Study the drawing (mm; zero at the part's minimum x, y, z) and answer. A direction names the side the tool comes from. Give positions to 0.01 mm unless a question says otherwise; leave off trailing zeros. Order: outer loops, then holes, each group sorted by start corner. A loop starts at its lowest first (then second) coordinate and runs counter-clockwise, first axis right, second up. Notation, with made-up numbers: (84.25, 41.5) - (134.25, 41.5) arc R8 ccw to (134.25, 46.5) - close; hole circle Ø4 at (53.25, 5.25). An arc over 180 degrees is marked (long way). Return JSON: item names as keys, results as strings.
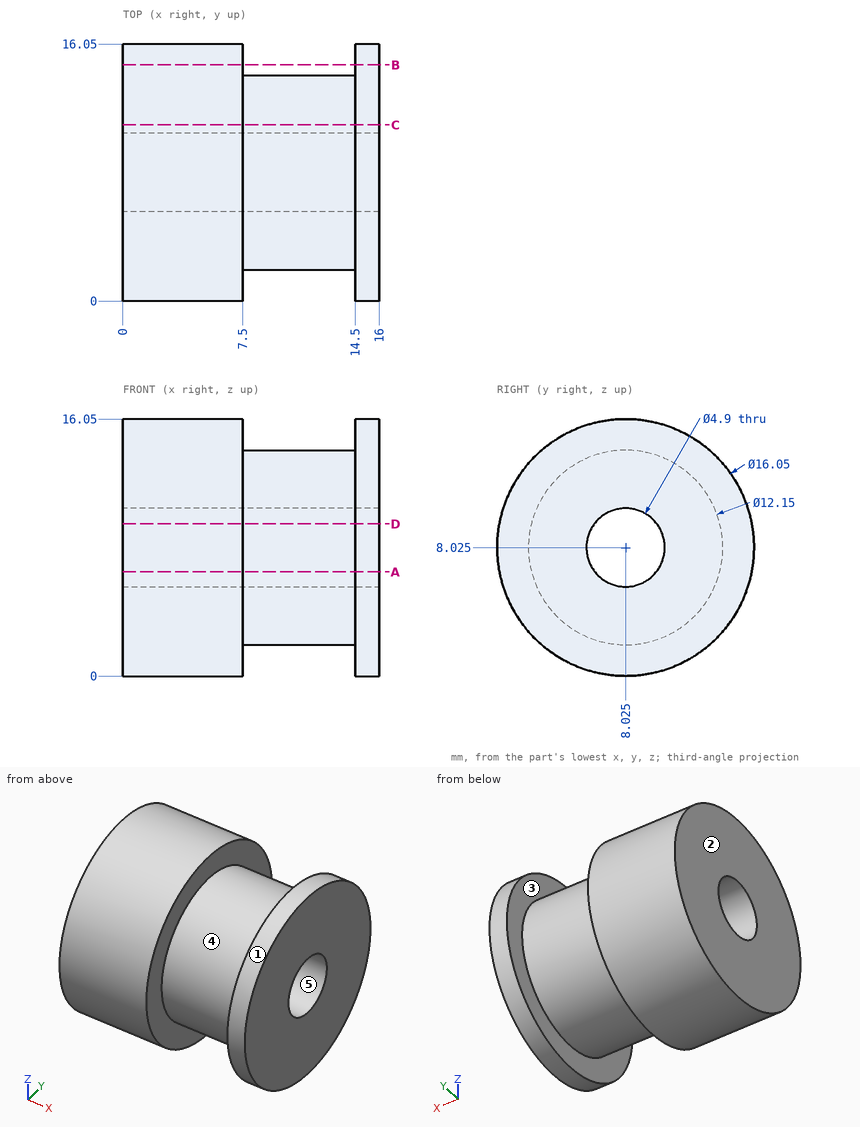
Q1. A cutting plane is placed at A-A (z = 6.5). Write down the section's boundary in (x, y).
Values:
{"outline": "(0, 0.15) - (7.5, 0.15) - (7.5, 2.14) - (14.5, 2.14) - (14.5, 0.15) - (16, 0.15) - (16, 6.11) - (0, 6.11) - close; (0, 9.94) - (16, 9.94) - (16, 15.9) - (14.5, 15.9) - (14.5, 13.91) - (7.5, 13.91) - (7.5, 15.9) - (0, 15.9) - close"}
Q2. A cutting plane is placed at C-C (y = 11). Write down the section's boundary in (x, z).
Values:
{"outline": "(0, 0.57) - (7.5, 0.57) - (7.5, 2.73) - (14.5, 2.73) - (14.5, 0.57) - (16, 0.57) - (16, 15.48) - (14.5, 15.48) - (14.5, 13.32) - (7.5, 13.32) - (7.5, 15.48) - (0, 15.48) - close"}
Q3. Determine the mould class of the marked faces 1, 2 and 3 for opening direction X: released by +X, released by -X, zero draft, split by the parting line, or undercut.
Values:
{"face 1": "zero draft", "face 2": "released by -X", "face 3": "undercut"}
Q4. A cutting plane is placed at B-B (y = 14.75). Write down the section's boundary in (x, z).
Values:
{"outline": "(0, 3.65) - (7.5, 3.65) - (7.5, 12.4) - (0, 12.4) - close; (14.5, 3.65) - (16, 3.65) - (16, 12.4) - (14.5, 12.4) - close"}
Q5. Given pin 1 (1 mm diameter, centred on x = 6.5, y = 2.5, fed in from -Z); pin 2 (3 mm diameter, centred on x = 14, y = 5.5, fed in from -Z); pin 3 (1.5 mm diameter, centred on x = 2, z = 2, fed in from -Y), each flat-ended and moving along its own axis, determine where each tip first touches the part or whether it passes through.
Values:
{"pin 1": "stops at z = 1.77", "pin 2": "stops at z = 0.08", "pin 3": "stops at y = 1.98"}
Q6. Consider L1, parallel to X at y = 14, z = 12.75; L2, parallel to Y at x = 11.25, z = 10; L3, parallel to Z at x = 10, y = 10.25. Determine where each line is inside the solid, lowest interval first.
Values:
{"L1": "x = 0 to 7.5, 14.5 to 16", "L2": "y = 2.28 to 6.58, 9.47 to 13.77", "L3": "z = 2.37 to 7, 9.05 to 13.68"}
Q7. A cutting plane is placed at D-D (z = 9.5). Write down the section's boundary in (x, y).
Values:
{"outline": "(0, 0.14) - (7.5, 0.14) - (7.5, 2.13) - (14.5, 2.13) - (14.5, 0.14) - (16, 0.14) - (16, 6.07) - (0, 6.07) - close; (0, 9.98) - (16, 9.98) - (16, 15.91) - (14.5, 15.91) - (14.5, 13.92) - (7.5, 13.92) - (7.5, 15.91) - (0, 15.91) - close"}
Q8. For the marked faces 4 and 5, determine the directions among +Z, -Z, +X, -X, +Y, -Y from which every point of the face is accessible in a straight line to the end or side of a thin tool.
Values:
{"face 4": "none", "face 5": "+X, -X"}
